Read the model definition and answer for the solid it produces. Units are mm, in the model's axes. A direction names the side the tool comes from. Coordinates: 2 decimals unless noted, no trailing zeros. Order: outer loops, then holes, each group sorted by start corner. A loop starts at its lowest first (then second) coordinate and runs counter-clockwise, first axis right, second up. Notation, with made-up numbers: (-9, 20) - (18, 20) arc R21 cw to (18, 55) - close; hole circle Ø5 at (-39, 58). An arc over 180 degrees is marked (long way). Write item = value, one per line.
Autodesk Inventor part; units mm, degrees
ref_plane "YZ Plane" through (0, 0, 0) normal (1, 0, 0) x (0, 1, 0)
ref_plane "XZ Plane" through (0, 0, 0) normal (0, 1, 0) x (-1, 0, 0)
ref_plane "XY Plane" through (0, 0, 0) normal (0, 0, 1) x (1, 0, 0)
sketch "Szkic1" plane through (0, 0, 0) normal (0, 1, 0) x (-1, 0, 0)
  circle A0 centre (0, 0) radius 5.5
  dimension "d0" = 11
extrude "Wyciągnięcie proste1" add sketch "Szkic1" along normal blind 10
sketch "Szkic2" plane through (0, 10, 0) normal (0, 1, 0) x (1, 0, 0)
  circle A0 centre (0, 0) radius 11
  dimension "d3" = 22
extrude "Wyciągnięcie proste2" add sketch "Szkic2" along normal blind 3
sketch "Szkic3" plane through (0, 13, 0) normal (0, 1, 0) x (1, 0, 0)
  point P0 (0, 0)
  point P1 (-8, 0)
  point P2 (0, -8)
  point P3 (8, 0)
  point P4 (0, 8)
  dimension "d6" = 8
  dimension "d9" = 360
hole "Otwór1" at (-8, 13, 0) at (0, 13, 8) at (8, 13, 0) at (0, 13, -8) direction (0, -1, 0) diameter 3 end through all
sketch "Szkic4" plane through (0, 13, 0) normal (0, 1, 0) x (1, 0, 0)
  point P0 (0, 0)
  point P1 (0, 0)
hole "Otwór2" at (0, 13, 0) direction (0, -1, 0) diameter 8 end through all
chamfer "Faza1" distance 0.5 angle 45 2 edges at (-11, 13, 0) (5.5, 0, 0)
thread "Gwint1"
properties part number "25_nakrętka trapezowa" material "Mosiądz, miękki żółty"
1) The part is cut by section D-D (y = 3.25). Determine the outline of the cut face in (x, z).
Returned:
outline = circle Ø11 at (0, 0); hole circle Ø8 at (0, 0)
2) Determine the mould class of faces 1 (the face through (5, 13, 0)), 2 (the face through (-6.536, 11.479, -0.325)), 3 (the face through (-2.38, 11.23, -10.74)) for opening direction X: pulls with the +X half, pulls with the -X half, needs draft (parallel to the pull), parting line crosses it, or undercut.
Returned:
face_1 = needs draft
face_2 = undercut
face_3 = parting line crosses it
3) The part is cut by section C-C (y = 11.5). Determine the outline of the cut face in (x, z).
Returned:
outline = circle Ø22 at (0, 0); hole circle Ø3 at (-8, 0); hole circle Ø8 at (0, 0); hole circle Ø3 at (0, -8); hole circle Ø3 at (0, 8); hole circle Ø3 at (8, 0)
4) Straight lines are drawn through the part: line 1 along Z through (x, y) = (0, 12.25); line 2 along X through (y, z) = (12, -0.75). For each, find the intervals that lie inside material, in ascending order. Write a range as from..to.
Returned:
line_1 = -11..-9.5, -6.5..-4, 4..6.5, 9.5..11
line_2 = -10.97..-9.3, -6.7..-3.93, 3.93..6.7, 9.3..10.97
5) The part is cut by section A-A (z = 0). Determine the outline of the cut face in (x, y), and give its area (3 significant figures).
Returned:
outline = (-11, 10) - (-9.5, 10) - (-9.5, 13) - (-10.5, 13) - (-11, 12.5) - close; (-6.5, 10) - (-5.5, 10) - (-5.5, 0.5) - (-5, 0) - (-4, 0) - (-4, 13) - (-6.5, 13) - close; (4, 0) - (5, 0) - (5.5, 0.5) - (5.5, 10) - (6.5, 10) - (6.5, 13) - (4, 13) - close; (9.5, 10) - (11, 10) - (11, 12.5) - (10.5, 13) - (9.5, 13) - close
area = 53.5 mm^2
6) For faces 4 (the face through (1.19, 5.18, 5.37)), 5 (the face through (3.905, 6.409, -0.867)), determine the directions among +Z, -Z, +X, -X, +Y, -Y from which every point of the face is accessible in a straight line to the end or side of a thin tool.
Returned:
face_4 = -Y
face_5 = +Y, -Y
7) The part is cut by section B-B (x = 0). Determine the outline of the cut face in (y, z).
Returned:
outline = (0, -5) - (0.5, -5.5) - (10, -5.5) - (10, -6.5) - (13, -6.5) - (13, -4) - (0, -4) - close; (0, 4) - (13, 4) - (13, 6.5) - (10, 6.5) - (10, 5.5) - (0.5, 5.5) - (0, 5) - close; (10, -11) - (12.5, -11) - (13, -10.5) - (13, -9.5) - (10, -9.5) - close; (10, 9.5) - (13, 9.5) - (13, 10.5) - (12.5, 11) - (10, 11) - close
8) Flat-ended cylindrical pins translate along their axes: pin 1 Ø1 at (y, z) = (4.5, -3.5) entering from +X; pin 2 Ø2 at (x, z) = (-1.5, -6.5) entering from -Y; pin 3 Ø1.5 at (x, z) = (5, -3.5) entering from -Y. Find the tip coordinate at first contact, or state that the pin passes through.
Returned:
pin_1 = 4.61
pin_2 = 10
pin_3 = 0.35
